from build123d import *

# Parameters (mm, degrees)
F1_DEPTH  = 76.2
F2_T      = -6.35
F3_W      = 76.2
F3_H      = 50.8
F3_H_2    = 10.16
F4_DEPTH  = 6.35
F6_DEPTH  = 76.2
F7_R      = 3.937
F7_R_2    = 1.905
F8_DEPTH  = 25.4
F9_W      = 63.5
F9_H      = 38.89375
F10_DEPTH = 3.175
F11_W     = 63.5
F11_H     = 37.67111
F12_DEPTH = 0.0762


with BuildPart() as f1:
    # F0 (on Right) → F1 (new body)
    with BuildSketch(Plane.YZ):
        Polygon((-34.085404, 0), (0, 0), (16.714596, 0), (-27.735404, 50.8), (-34.085404, 50.8), align=None)
    extrude(amount=F1_DEPTH)

    # F2
    f2_openings = [f1.faces().sort_by_distance(p)[0] for p in [
        (38.1, -5.510404, 25.4),
    ]]
    offset(amount=F2_T, openings=f2_openings)

    # F3 (on face) → F4 (join)
    with BuildSketch(Plane(origin=(0, 0, 0), x_dir=(1, 0, 0), z_dir=(0, 0, -1))):
        with Locations((38.1, 8.685404)):
            Rectangle(F3_W, F3_H)
        with Locations((38.1, -21.794596)):
            Rectangle(F3_W, F3_H_2)
    extrude(amount=-F4_DEPTH)

    # F5 (on face) → F6 (cut)
    with BuildSketch(Plane.YZ.offset(76.2)):
        with BuildLine():
            Line((26.874596, 6.35), (11.158346, 6.35))
            ThreePointArc((11.158346, 6.35), (18.798291, 2.635004), (26.874596, 0))
            Line((26.874596, 0), (26.874596, 6.35))
        make_face()
    extrude(amount=-F6_DEPTH, mode=Mode.SUBTRACT)

    # F7 (on face) → F8 (cut)
    with BuildSketch(Plane.XZ.offset(34.085404)):
        with Locations((38.1, 25.4)):
            Circle(F7_R)
        with Locations((38.1, 33.274)):
            Circle(F7_R_2)
        with Locations((38.1, 17.526)):
            Circle(F7_R_2)
        with Locations((30.226, 25.4)):
            Circle(F7_R_2)
        with Locations((45.974, 25.4)):
            Circle(F7_R_2)
    extrude(amount=-F8_DEPTH, mode=Mode.SUBTRACT)

    # F9 (on face) → F10 (cut)
    with BuildSketch(Plane.XY.offset(6.35)):
        with Locations((38.1, -8.288529)):
            Rectangle(F9_W, F9_H)
    extrude(amount=-F10_DEPTH, mode=Mode.SUBTRACT)

    # F11 (on face) → F12 (cut)
    with BuildSketch(Plane(origin=(0, -27.735404, 0), x_dir=(-1, 0, 0), z_dir=(0, 1, 0))):
        with Locations((-38.1, 25.614445)):
            Rectangle(F11_W, F11_H)
    extrude(amount=-F12_DEPTH, mode=Mode.SUBTRACT)


solid = f1.part
Could you check a few things on this model? Use its own coordinates, in mm. A direction names the side the tool comes from. Give positions to 0.01 mm unless a question says otherwise; leave off trailing zeros. Loops run counter-clockwise (first coordinate to the right, second up) from the corner with the lowest first, then second, coordinate; pieces in that order, holes last. Notation, with made-up numbers: (78, -18.5) -> (84, -18.5) arc R24 cw to (84, -3.5) -> close; hole circle Ø7 at (-25, -2.5). An arc over 180 degrees is marked (long way). Answer as CSV lines item,"result". Start each with the question number.
(1) Which directions (+Z, -Z, +X, -X, +Y, -Y) give clear straight access to the entire face, cutting with the end or side of a thin tool? Please do faces 1 (the flat face through (39, -27.812, 30)), 2 (the flat face through (69.85, -13, 20)), 3 (the flat face through (38, -31, 50.8)), 4 (the flat face through (38, 11.158, 5)).
(2) If we section it at B-B on y = -29.5: Write out the boundary of the cut face in (x, z) (3 decimals), then the cut area to 3 significant figures.
(3) I'm going to push flat-ended pins straight in: pin 1 Ø1.8 at (x, z) = (43, 5.5) entering from +Y; pin 2 Ø5 at (y, z) = (-13.5, 40.5) entering from -X; pin 3 Ø4 at (x, y) = (65, -18) entering from +Z (3 decimals); pin 4 Ø8 at (x, y) = (13, 15.5) entering from +Z. Where does each tip first touch, or does it pass through?
(4) We'd pull the mould along Y, two halves only. Please class faces 5 (the flat face through (6.35, -13, 20)), 6 (the cylindrical face through (38.979, -30.992, 31.584)), 7 (the flat face through (38, -34.085, 20)): released by +Y, released by -Y, zero draft, split by the parting line, or undercut.
(5) If we section it at C-C on z = 25.4: Write out the boundary of the cut face in (x, y).
(6) If we section it at D-D on x = 24.5: Write out the boundary of the cut face in (y, z) (3 decimals).
(7) If we section it at A-A on x = 38.1: Write out the boundary of the cut face in (y, z) (3 decimals), then the cut area to 3 significant figures.
(8) I need wall thicknesses on probe 1 along Z at (x, y) = (38.1, -32.5); probe 2 along X at (y, z) = (-13.5, 11.5). Which ranges of each line are inside material? Lowest first, please.
Computed:
1,face 1,"+Y"
1,face 2,"none"
1,face 3,"+Z, +X, -X, +Y, -Y"
1,face 4,"+Z"
2,outline,"(0, 0) -> (76.2, 0) -> (76.2, 50.8) -> (0, 50.8) -> close; hole circle Ø3.81 at (30.226, 25.4); hole circle Ø7.874 at (38.1, 25.4); hole circle Ø3.81 at (38.1, 17.526); hole circle Ø3.81 at (38.1, 33.274); hole circle Ø3.81 at (45.974, 25.4)"
2,area,"3,780 mm2"
3,pin 1,"stops at y = 14.43"
3,pin 2,"passes through"
3,pin 3,"stops at z = 3.175"
3,pin 4,"stops at z = 6.16"
4,face 5,"undercut"
4,face 6,"zero draft"
4,face 7,"released by -Y"
5,outline,"(0, -34.09) -> (28.32, -34.09) -> (28.32, -27.81) -> (6.35, -27.81) -> (6.35, -5.51) -> (0, -5.51) -> close; (32.13, -34.09) -> (34.16, -34.09) -> (34.16, -27.81) -> (32.13, -27.81) -> close; (42.04, -34.09) -> (44.07, -34.09) -> (44.07, -27.81) -> (42.04, -27.81) -> close; (47.88, -34.09) -> (76.2, -34.09) -> (76.2, -5.51) -> (69.85, -5.51) -> (69.85, -27.81) -> (47.88, -27.81) -> close"
6,outline,"(-34.085, 0) -> (26.875, 0) arc R61.958 cw to (11.158, 6.35) -> (11.158, 3.175) -> (-27.735, 3.175) -> (-27.735, 6.779) -> (-27.812, 6.779) -> (-27.812, 44.45) -> (-22.179, 44.45) -> (-27.735, 50.8) -> (-34.085, 50.8) -> close"
7,outline,"(-34.085, 0) -> (26.875, 0) arc R61.958 cw to (11.158, 6.35) -> (11.158, 3.175) -> (-27.735, 3.175) -> (-27.735, 6.779) -> (-27.812, 6.779) -> (-27.812, 15.621) -> (-34.085, 15.621) -> close; (-34.085, 19.431) -> (-27.812, 19.431) -> (-27.812, 21.463) -> (-34.085, 21.463) -> close; (-34.085, 29.337) -> (-27.812, 29.337) -> (-27.812, 31.369) -> (-34.085, 31.369) -> close; (-34.085, 35.179) -> (-27.812, 35.179) -> (-27.812, 44.45) -> (-22.179, 44.45) -> (-27.735, 50.8) -> (-34.085, 50.8) -> close"
7,area,"407 mm2"
8,probe 1,"z = 0 to 15.62, 19.43 to 21.46, 29.34 to 31.37, 35.18 to 50.8"
8,probe 2,"x = 0 to 6.35, 69.85 to 76.2"
